The figure shows three views and two pictorial views of one solid part (mm, origin at its lowest corner). Answer the questions. A direction names the side the tool comes from. Coordinates: 2 decimals unless noted, no trailing zeros. Write each loop counter-clockwise with the first axis right and the second up, starting at its lowest first coordinate (ties: lowest second). Pieces come first, ordered by that corner, then holes. Notation, with made-up numbers: M 28,39.25 L 42,39.25 A30 cw 42,76.25 Z; hole C 18,26 d9. An arc over 180 degrees is marked long. Answer as CSV lines item,"result".
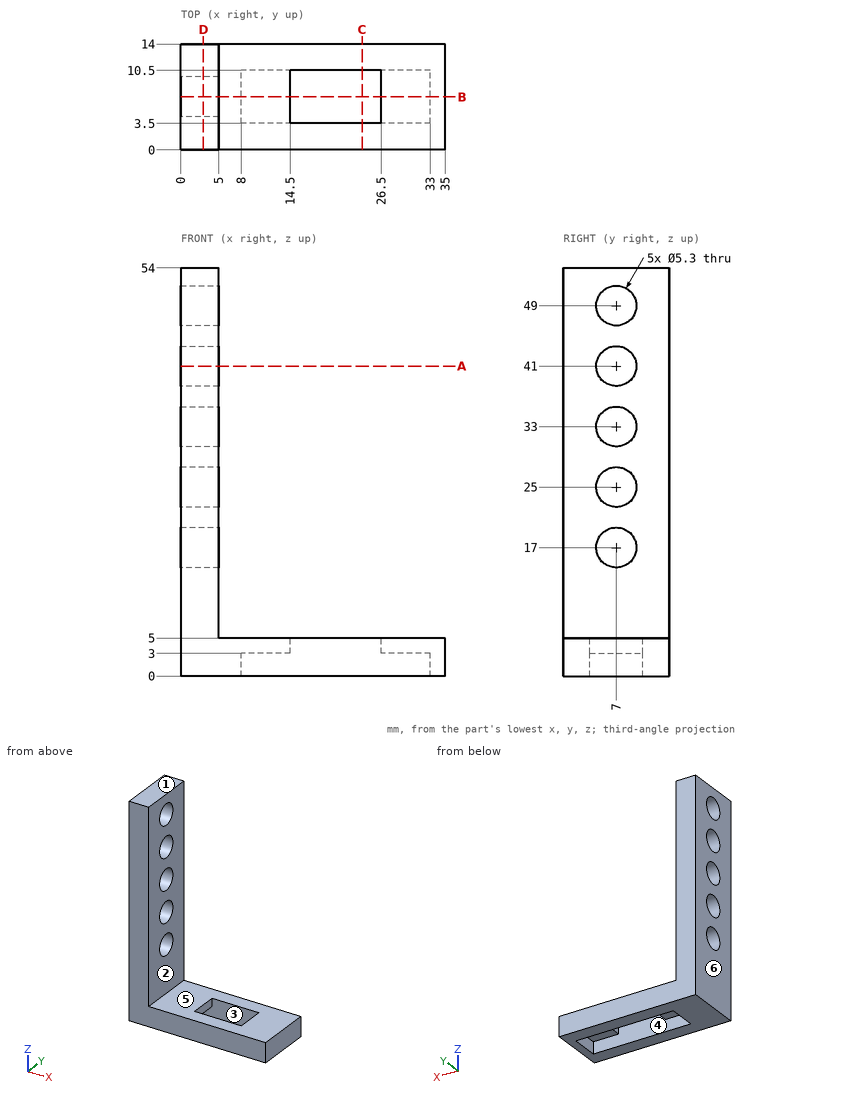
Q1. Straight lines are drawn through the part: line 1 (Y direction, x = 2.3, z = 25); line 2 (Z direction, x = 4, y = 4.75); line 3 (Z direction, x = 12.5, y = 6.5). For each, find the intervals that lie inside material, in ascending order.
Output:
line 1,"0 to 4.35, 9.65 to 14"
line 2,"0 to 15.6, 18.4 to 23.6, 26.4 to 31.6, 34.4 to 39.6, 42.4 to 47.6, 50.4 to 54"
line 3,"3 to 5"
Q2. Flat-ended cylindrical pins translate along their axes: pin 1 Ø7 at (y, z) = (6, 35) entering from +X; pin 2 Ø5 at (x, y) = (30, 7) entering from -Z. Find the tip coordinate at first contact, or state that the pin passes through.
Output:
pin 1,"x = 5"
pin 2,"z = 3"
Q3. Find section A-A (z = 41). Give the vertices of the cut face in (x, y).
Output:
outline,"M 0,0 L 5,0 L 5,4.35 L 0,4.35 Z; M 0,9.65 L 5,9.65 L 5,14 L 0,14 Z"
Q4. The mould has two halves that part along X. Classify the marked faces 3, 4, 5 and 6: pulls with the +X half, pulls with the -X half, needs draft (parallel to the pull), parting line crosses it, or undercut.
Output:
face 3,"undercut"
face 4,"undercut"
face 5,"needs draft"
face 6,"pulls with the -X half"
Q5. Find section B-B (y = 7). Count the separate pieces of the cut face and the enclosed holes in it, and give its area (4 significant figures).
Output:
separate pieces,"7"
enclosed holes,"0"
area,"188.5 mm2"
Q6. Find section D-D (x = 3). Give the vertices of the cut face in (y, z), and give its area (3 significant figures).
Output:
outline,"M 0,0 L 14,0 L 14,54 L 0,54 Z; hole C 7,17 d5.3; hole C 7,25 d5.3; hole C 7,33 d5.3; hole C 7,41 d5.3; hole C 7,49 d5.3"
area,"646 mm2"
Q7. Find section C-C (x = 24). Give the vertices of the cut face in (y, z).
Output:
outline,"M 0,0 L 3.5,0 L 3.5,5 L 0,5 Z; M 10.5,0 L 14,0 L 14,5 L 10.5,5 Z"
Q8. For the marked faces 1 and 2, determine the directions among +Z, -Z, +X, -X, +Y, -Y from which every point of the face is accessible in a straight line to the end or side of a thin tool.
Output:
face 1,"+Z, +X, -X, +Y, -Y"
face 2,"+Z, +X, +Y, -Y"
